from build123d import *

# Parameters (mm, degrees)
F2_R            = 12.5
F3_DEPTH        = 20.001
F3_COPIES_COUNT = 6


# Not quite as in the source:
# - a pattern or mirror of a feature is missing from the dataset's text; its kind, count and spacing are read off the source's solid


with BuildPart() as f1:
    # F0 (on Front) → F1 (revolve)
    with BuildSketch(Plane.XZ):
        Polygon((-100, 37.5), (0, 37.5), (0, 90), (-20, 90), (-20, 47.5), (-100, 47.5), align=None)
    revolve(axis=Axis((-107.4553492388, 0, 0), (-1, 0, 0)))

    # F2 (on face) → F3 (cut, through all)
    with BuildSketch(Plane(origin=(-20, 0, 0), x_dir=(0, -1, 0), z_dir=(-1, 0, 0))):
        with Locations((0, 70)):
            Circle(F2_R)
    f3 = extrude(amount=-F3_DEPTH, mode=Mode.SUBTRACT)

    # F3_copies: F3 ×6 about axis
    f3_copies_axis = Axis((0, 0, 0), (1, 0, 0))
    for i in range(1, F3_COPIES_COUNT):
        add(f3.rotate(f3_copies_axis, i * 360 / F3_COPIES_COUNT), mode=Mode.SUBTRACT)


solid = f1.part
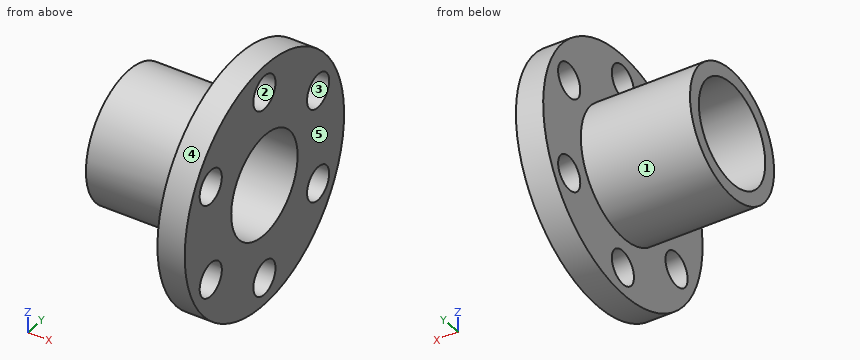
CAD build for the part. Positions are in the model's coordinates, mm. Face numbers are marked on the shaded views. A direction names the side the tool comes from. Coordinates: 2 decimals unless noted, no trailing zeros. Loops run counter-clockwise (first coordinate to the right, second up) from the corner with the lowest first, then second, coordinate; pieces in that order, holes last. Notation, with made-up numbers: (53.5, -20.75) - (78.5, -20.75) arc R18 ccw to (78.5, 9.25) - close; hole circle Ø7 at (27.25, 59.5). An arc over 180 degrees is marked (long way). Use one line per item in the form item = value. Start each with the question number.
1) Band-saw the part on A-A (z = 0). Give the cut face in (x, y).
2) Band-saw the part on B-B (y = 0). Give the cut face in (x, z), and give its area (3 significant figures).
3) Two-plate mould, pull along Y, no slides. Class the marked faces 3, 4 and 5: +Y half, -Y half, draft (parallel to the pull), parting line (faces both ways), or undercut.
4) Band-saw the part on D-D (x = -46.5). Give the cut face in (y, z).
5) Flat gauge pins, fed straight in: pin 1 (10 mm diameter, centred on x = -68.5, y = 38, fed in from -Z); pin 2 (10 mm diameter, centred on x = -36, y = 54, fed in from -Z); pin 3 (12 mm diameter, centred on x = -70, y = -47.5, fed in from +Z); pin 4 (8 mm diameter, centred on x = -76, z = -14, fed in from -Y). Where does each tip first touch, or does it go through?
6) Drill centre lines: L1, parallel to Z at x = -31, y = -17; L2, parallel to Y at x = -49, z = 0; L3, parallel to Z at x = -19, y = 63.5. Where is each one in solid material? Low to high. Write a range as from..to.
7) Band-saw the part on C-C (z = 32.5). Give the cut face in (x, y).
8) Tool access for the marked faces 1 and 2: list every direction of +Z, -Z, +X, -X, +Y, -Y with a clear straight run to the whole face (end or side of a thin tool).
Check values:
q1.outline = (-100, -47.5) - (-20, -47.5) - (-20, -90) - (0, -90) - (0, -37.5) - (-100, -37.5) - close; (-100, 37.5) - (0, 37.5) - (0, 90) - (-20, 90) - (-20, 47.5) - (-100, 47.5) - close
q2.outline = (-100, -47.5) - (-20, -47.5) - (-20, -57.5) - (0, -57.5) - (0, -37.5) - (-100, -37.5) - close; (-100, 37.5) - (0, 37.5) - (0, 57.5) - (-20, 57.5) - (-20, 47.5) - (-100, 47.5) - close; (-20, -90) - (0, -90) - (0, -82.5) - (-20, -82.5) - close; (-20, 82.5) - (0, 82.5) - (0, 90) - (-20, 90) - close
q2.area = 2,700 mm2
q3.face_3 = undercut
q3.face_4 = parting line
q3.face_5 = draft
q4.outline = circle Ø95 at (0, 0); hole circle Ø75 at (0, 0)
q5.pin_1 = -34.17
q5.pin_2 = through
q5.pin_3 = 23.11
q5.pin_4 = -46.44
q6.L1 = -44.35..-33.43, 33.43..44.35
q6.L2 = -47.5..-37.5, 37.5..47.5
q6.L3 = -63.78..-47.16, -22.84..22.84, 47.16..63.78
q7.outline = (-100, -34.64) - (-20, -34.64) - (-20, -48.37) - (0, -48.37) - (0, -18.71) - (-100, -18.71) - close; (-100, 18.71) - (0, 18.71) - (0, 48.37) - (-20, 48.37) - (-20, 34.64) - (-100, 34.64) - close; (-20, -83.93) - (0, -83.93) - (0, -72.87) - (-20, -72.87) - close; (-20, 72.87) - (0, 72.87) - (0, 83.93) - (-20, 83.93) - close
q8.face_1 = -X
q8.face_2 = +X, -X
